from build123d import *

# Parameters (mm, degrees)
SKETCH1_R           = 31
SKETCH1_R_2         = 15
BOSS_EXTRUDE2_DEPTH = 8
SKETCH4_R           = 28
SKETCH4_R_2         = 20
CUT_EXTRUDE2_DEPTH  = 0.1


with BuildPart() as part:
    # Sketch1 → Boss-Extrude2 (new body)
    with BuildSketch(Plane(origin=(0, 0, 0), x_dir=(1, 0, 0), z_dir=(0, 1, 0))):
        with Locations(Location((0, 0, 0), (0, 0, 270))):
            Circle(SKETCH1_R)
        with Locations(Location((0, 0, 0), (0, 0, 270))):
            Circle(SKETCH1_R_2, mode=Mode.SUBTRACT)
    boss_extrude2 = extrude(amount=BOSS_EXTRUDE2_DEPTH)

    # Sketch4 → Cut-Extrude2 (cut)
    with BuildSketch(Plane(origin=(0, 8, 0), x_dir=(1, 0, 0), z_dir=(0, 1, 0))):
        with Locations(Location((0, 0, 0), (0, 0, 270))):
            Circle(SKETCH4_R)
        with Locations(Location((0, 0, 0), (0, 0, 270))):
            Circle(SKETCH4_R_2, mode=Mode.SUBTRACT)
    cut_extrude2 = extrude(amount=-CUT_EXTRUDE2_DEPTH, mode=Mode.SUBTRACT)


with BuildPart() as mirror2_1:
    # Mirror2: Boss-Extrude2 across Top Plane
    add(boss_extrude2.mirror(Plane(origin=(0, 0, 0), x_dir=(1, 0, 0), z_dir=(0, 1, 0))))

    # Mirror2 2: Cut-Extrude2 across Top Plane
    add(cut_extrude2.mirror(Plane(origin=(0, 0, 0), x_dir=(1, 0, 0), z_dir=(0, 1, 0))), mode=Mode.SUBTRACT)


with BuildPart() as part_1:
    add(part.part)

    # Mirror2 united with what the copies touc: union Mirror2_1
    add(mirror2_1.part)


solid = part_1.part
Geometry check sheet. Reference: the model listing, model coordinates, mm. Give positions to 0.01 mm unless a question says otherwise; leave off trailing zeros. Write each loop counter-clockwise with the first axis right and the second up, starting at its lowest first coordinate (ties: lowest second). Pieces come first, ordered by that corner, then holes.
1) Cross-section at B-B (x = 0). Record the boundary of the cut face in (y, z).
Values follow:
outline: (-8, -31) - (8, -31) - (8, -28) - (7.9, -28) - (7.9, -20) - (8, -20) - (8, -15) - (-8, -15) - (-8, -20) - (-7.9, -20) - (-7.9, -28) - (-8, -28) - close; (-8, 15) - (8, 15) - (8, 20) - (7.9, 20) - (7.9, 28) - (8, 28) - (8, 31) - (-8, 31) - (-8, 28) - (-7.9, 28) - (-7.9, 20) - (-8, 20) - close
2) Cross-section at D-D (x = -23). Record the boundary of the cut face in (y, z), plus the area to 3 significant figures.
Values follow:
outline: (-8, -20.78) - (8, -20.78) - (8, -15.97) - (7.9, -15.97) - (7.9, 15.97) - (8, 15.97) - (8, 20.78) - (-8, 20.78) - (-8, 15.97) - (-7.9, 15.97) - (-7.9, -15.97) - (-8, -15.97) - close
area: 659 mm2
3) Thickness scan on line 1 (X direction, y = 7.95, z = 0); line 2 (X direction, y = 0.25, z = 0); line 3 (X direction, y = 5, z = -10). Record the ranges inside material, lowest first.
Values follow:
line 1: x = -31 to -28, -20 to -15, 15 to 20, 28 to 31
line 2: x = -31 to -15, 15 to 31
line 3: x = -29.34 to -11.18, 11.18 to 29.34
4) Cross-section at C-C (y = 1.25). Record the boundary of the cut face in (x, z).
Values follow:
outline: circle Ø62 at (0, 0); hole circle Ø30 at (0, 0)
5) Cross-section at A-A (z = 0). Record the boundary of the cut face in (x, y).
Values follow:
outline: (-31, -8) - (-28, -8) - (-28, -7.9) - (-20, -7.9) - (-20, -8) - (-15, -8) - (-15, 8) - (-20, 8) - (-20, 7.9) - (-28, 7.9) - (-28, 8) - (-31, 8) - close; (15, -8) - (20, -8) - (20, -7.9) - (28, -7.9) - (28, -8) - (31, -8) - (31, 8) - (28, 8) - (28, 7.9) - (20, 7.9) - (20, 8) - (15, 8) - close
6) Go/stop test with flat-tipped pins: pin 1 Ø1.5 at (y, z) = (1.5, 24) entering from +X; pin 2 Ø6 at (y, z) = (6, 21) entering from -X; pin 3 Ø4 at (x, y) = (8.5, 1) entering from +Z. Record where each tip stops, or that it passes through.
Values follow:
pin 1: stops at x = 20.5
pin 2: stops at x = -25.24
pin 3: stops at z = 30.31
7) Release check for a two-part mould opening along Z. For faces 1 (the face through (19, -7.9, -7)), 2 (the face through (-27.4, 8, -7)), 3 (the face through (30.736, 0.112, -4.036)), 4 (the face through (19, 7.9, -7)) record: released by +Z, released by -Z, zero draft, split by the parting line, or undercut.
Values follow:
face 1: undercut
face 2: zero draft
face 3: split by the parting line
face 4: undercut
